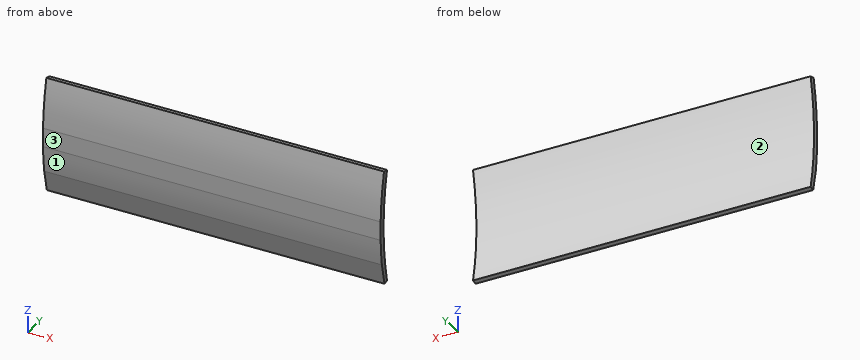
Autodesk Inventor part; units mm, degrees
ref_plane "YZ Plane" through (0, 0, 0) normal (1, 0, 0) x (0, 1, 0)
ref_plane "XZ Plane" through (0, 0, 0) normal (0, 1, 0) x (-1, 0, 0)
ref_plane "XY Plane" through (0, 0, 0) normal (0, 0, 1) x (1, 0, 0)
sketch "スケッチ1" plane through (0, 0, 0) normal (1, 0, 0) x (0, 1, 0)
  arc A0 (6.2855, 30) -> (6.2855, -30) centre (141.6068, 0) ccw
  arc A1 (3.3566, 30.6493) -> (3.3566, -30.6493) centre (141.6068, 0) ccw
  line L0 (6.2855, 30) -> (3.3566, 30.6493)
  line L1 (6.2855, -30) -> (3.3566, -30.6493)
  line L2 (0, -42.909) -> (0, 42.909)
  point P0 (0, 0)
  point P1 (0, 0)
  dimension "d0" = 3
  dimension "d1" = 60
  dimension "d2" = 25
extrude "押し出し1" add sketch "スケッチ1" along normal blind 180
sketch "スケッチ2" plane through (0, 0, 0) normal (-1, 0, 0) x (0, 0, 1)
  arc A0 (-30.6493, 3.3566) -> (30.6493, 3.3566) centre (0, 141.6068) ccw
  line L0 (-30.6493, 3.3566) -> (-6.3173, -2.0376)
  line L1 (-30.6493, 3.3566) -> (-30, 6.2855)
  line L2 (-30.5411, 3.8448) -> (-18.9336, 1.2715)
  point P0 (0, 0)
  dimension "d5" = 0.5
extrude "押し出し2" cut sketch "スケッチ2" against normal through all
sketch "スケッチ3" plane through (0, 0, 0) normal (-1, 0, 0) x (0, 0, 1)
  line L0 (-5, 0.0883) -> (5, 0.0883)
  arc A0 (-18.9336, 1.2715) -> (30.6493, 3.3566) centre (0, 141.6068) ccw
  point P0 (0, 0)
  dimension "d9" = 10
extrude "押し出し3" cut sketch "スケッチ3" against normal through all
properties part number "element_2" material "CFRP"
Can you work these out from the model? Positions are in its coordinate system, mm. Face numbers are marked on the shaded views. Round coordinates to 2 decimals unless told otherwise and drop trailing zeros. Order: outer loops, then holes, each group sorted by start corner. A loop starts at its lowest first (then second) coordinate and runs counter-clockwise, first axis right, second up. Notation, with made-up numbers: M 6,18.25 L 40,18.25 A33 ccw 40,46.25 Z; hole C 6.25,-23 d3. An arc over 180 degrees is marked long. Use a Markdown table: item, result.
1) I'm going to push a flat-ended pin straight in: P1, Ø8, axis at x = 50, z = -21, coming from the -Y side. Where does the tip first touch, or does it pass through?
Geometry says:
| item | result |
|---|---|
| P1 | stops at y = 1.02 |
2) Imagine slicing it at B-B (z = 12). List the corners of the cut face in (x, y) for me, then the cut area to 3 significant figures.
Geometry says:
| item | result |
|---|---|
| outline | M 0,0.51 L 180,0.51 L 180,3.52 L 0,3.52 Z |
| area | 542 mm² |
3) If we mould it in two halves opening along Z, with no side actions, what happens to the marked faces 1, 2 and 3? For each: +Z half, -Z half, draft (parallel to the pull), parting line (faces both ways), or undercut.
Geometry says:
| item | result |
|---|---|
| face 1 | -Z half |
| face 2 | undercut |
| face 3 | draft |
4) Imagine slicing it at C-C (z = 26.5). List the corners of the cut face in (x, y) for me.
Geometry says:
| item | result |
|---|---|
| outline | M 0,2.5 L 180,2.5 L 180,5.56 L 0,5.56 Z |
5) If I drill on line 1 along Y through (x, z) = (75, -16.5); line 2 along Y through (x, z) = (116, 3.5), over which ranges is the centre line in solid material (lowest first)?
Geometry says:
| item | result |
|---|---|
| line 1 | y = 0.96 to 3.99 |
| line 2 | y = 0.09 to 3.04 |
6) Imagine slicing it at A-A (x = 50). List the corners of the cut face in (y, z) for me, then the cut area to 3 significant figures.
Geometry says:
| item | result |
|---|---|
| outline | M 0.09,-5 A141.61 ccw 1.27,-18.93 L 3.84,-30.54 L 6.29,-30 A138.61 cw 6.29,30 L 3.36,30.65 A141.61 ccw 0.09,5 Z |
| area | 179 mm² |
